```python
from build123d import *

# Parameters (mm, degrees)
BOSS_EXTRUDE1_DEPTH = 4
SKETCH2_R           = 0.2
CUT_EXTRUDE1_DEPTH  = 8
FILLET2_R           = 0.4
FILLET1_R           = 0.6
FILLET3_R           = 2
BOSS_EXTRUDE2_DEPTH = 8
FILLET4_R           = 0.6
CUT_EXTRUDE2_DEPTH  = 0.5
CUT_EXTRUDE2_DRAFT  = -45
CHAMFER1_SIZE       = 0.3


with BuildPart() as part:
    # Sketch1 → Boss-Extrude1 (new, symmetric)
    with BuildSketch(Plane.XY):
        Polygon((0, 9), (6, 9), (6, 0), (7.5, 0), (7.5, -7), (10.5, -7), (10.5, 12), (0, 12), align=None)
    extrude(amount=BOSS_EXTRUDE1_DEPTH, both=True)

    # Sketch2 → Cut-Extrude1 (cut)
    with BuildSketch(Plane.XY.offset(4)):
        with Locations((7.5, -0.2)):
            Circle(SKETCH2_R)
    extrude(amount=-CUT_EXTRUDE1_DEPTH, mode=Mode.SUBTRACT)

    # Fillet2
    fillet2_edges = [part.edges().sort_by_distance(p)[0] for p in [
        (6, 0, 0),
        (7.5, -0.4, 0),
    ]]
    fillet(fillet2_edges, radius=FILLET2_R)

    # Fillet1
    fillet1_edges = [part.edges().sort_by_distance(p)[0] for p in [
        (10.5, -7, 0),
        (7.5, -7, 0),
        (6, 9, 0),
    ]]
    fillet(fillet1_edges, radius=FILLET1_R)

    # Fillet3
    fillet3_edges = [part.edges().sort_by_distance(p)[0] for p in [
        (10.5, 12, 0),
    ]]
    fillet(fillet3_edges, radius=FILLET3_R)

    # Mirror1: part across plane


with BuildPart() as part_1:
    add(part.part)
    add(part.part.mirror(Plane(origin=(0, 12, 4), x_dir=(0, 0, 1), z_dir=(1, 0, 0))))

    # Sketch3 → Boss-Extrude2 (add)
    with BuildSketch(Plane.XY.offset(4)):
        with BuildLine():
            Line((-8.1, -7), (-9.9, -7))
            ThreePointArc((-9.9, -7), (-10.324264069, -6.824264069), (-10.5, -6.4))
            Line((-10.5, -6.4), (-10.5, -10))
            Line((-10.5, -10), (-7.5, -10))
            Line((-7.5, -10), (-7.5, -6.4))
            ThreePointArc((-7.5, -6.4), (-7.675735931, -6.824264069), (-8.1, -7))
        make_face()
    extrude(amount=-BOSS_EXTRUDE2_DEPTH)

    # Fillet4
    fillet4_edges = [part_1.edges().sort_by_distance(p)[0] for p in [
        (-7.5, -10, 0),
    ]]
    fillet(fillet4_edges, radius=FILLET4_R)


with BuildPart() as cut_extrude2_tool:
    # Sketch4 → Cut-Extrude2 (with draft: the straight prism first)
    with BuildSketch(Plane(origin=(0, 12, 0), x_dir=(1, 0, 0), z_dir=(0, 1, 0))):
        Polygon((-2.5, -1.443375673), (2.5, -1.443375673), (0, 2.886751346), align=None)
    extrude(amount=-CUT_EXTRUDE2_DEPTH)
    # Cut-Extrude2: the draft: its side faces are tilted about the plane it starts from
    cut_extrude2_sides = [cut_extrude2_tool.faces().sort_by_distance(p)[0] for p in [
        (0, 11.75, 1.443375673),
        (1.25, 11.75, -0.721687836),
        (-1.25, 11.75, -0.721687836),
    ]]
    draft(cut_extrude2_sides, Plane(origin=(0, 12, 0), x_dir=(1, 0, 0), z_dir=(0, 1, 0)), CUT_EXTRUDE2_DRAFT)


with BuildPart() as part_2:
    add(part_1.part)

    # Cut-Extrude2: cut by cut_extrude2_tool
    add(cut_extrude2_tool.part, mode=Mode.SUBTRACT)

    # Chamfer1
    chamfer1_edges = [part_2.edges().sort_by_distance(p)[0] for p in [
        (-9.3, -10, 4),
        (0, 9, -4),
        (-9.3, -10, -4),
        (-7.675735931, -9.824264069, 4),
        (-7.675735931, -9.824264069, -4),
        (6.95, 0, -4),
        (6.95, 0, 4),
        (7.5, -3.523606798, -4),
        (7.686834472, -0.128635582, -4),
        (7.534851628, -0.483914279, -4),
        (6.117157288, 0.117157288, -4),
        (7.686834472, -0.128635582, 4),
        (7.5, -3.523606798, 4),
        (7.534851628, -0.483914279, 4),
        (6.117157288, 0.117157288, 4),
        (10.5, 1.8, -4),
        (10.5, 1.8, 4),
        (6, 4.4, -4),
        (9, -7, -4),
        (7.675735931, -6.824264069, -4),
        (10.324264069, -6.824264069, -4),
        (9, -7, 4),
        (6, 4.4, 4),
        (7.675735931, -6.824264069, 4),
        (10.324264069, -6.824264069, 4),
        (5.824264069, 8.824264069, -4),
        (5.824264069, 8.824264069, 4),
        (0, 12, -4),
        (0, 12, 4),
        (9.914213562, 11.414213562, -4),
        (9.914213562, 11.414213562, 4),
        (-6, 4.4, 4),
        (-6.95, 0, 4),
        (-7.5, -5.023606798, 4),
        (-10.5, 0, 4),
        (-7.686834472, -0.128635582, 4),
        (-6, 4.4, -4),
        (-6.95, 0, -4),
        (-7.5, -5.023606798, -4),
        (-10.5, 0, -4),
        (-7.686834472, -0.128635582, -4),
        (-6.117157288, 0.117157288, 4),
        (-6.117157288, 0.117157288, -4),
        (-7.534851628, -0.483914279, 4),
        (-7.534851628, -0.483914279, -4),
        (-5.824264069, 8.824264069, 4),
        (-5.824264069, 8.824264069, -4),
        (-9.914213562, 11.414213562, 4),
        (-9.914213562, 11.414213562, -4),
        (0, 9, 4),
    ]]
    chamfer(chamfer1_edges, length=CHAMFER1_SIZE)


solid = part_2.part
```
Could you check a few things on this model? Use its own coordinates, in mm. A direction names the side the tool comes from. Give positions to 0.01 mm unless a question says otherwise; leave off trailing zeros. Write each loop counter-clockwise with the first axis right and the second up, starting at its lowest first coordinate (ties: lowest second). Pieces come first, ordered by that corner, then holes. Notation, with made-up numbers: (-31, 28.5) -> (15, 28.5) arc R12 ccw to (15, 45.5) -> close; hole circle Ø1 at (72, -10.75). An arc over 180 degrees is marked (long way). Write each question's results on one line, items separated by ' | '.
1. Will these pins go through, and if not, where does the flat tip stop? pin 1 Ø2 at (x, z) = (8.5, 1) entering from -Y; pin 2 Ø5 at (x, y) = (-1.5, 4.5) entering from -Z; pin 3 Ø1.2 at (x, z) = (6.5, 0.5) entering from -Y; pin 4 Ø1.4 at (x, z) = (0.5, -0.5) entering from +Y.
Check sheet entries:
pin 1: stops at y = -7 | pin 2: passes through | pin 3: stops at y = 0 | pin 4: stops at y = 11.94
2. I need wall thicknesses on L1, parallel to X at y = -3.75, z = 2.25; L2, parallel to X at y = 6.5, z = -1.75; L3, parallel to Y at x = 4, z = -0.75. Which ranges of each line are inside material? Lowest first, please.
Check sheet entries:
L1: x = -10.5 to -7.5, 7.5 to 10.5 | L2: x = -10.5 to -6, 6 to 10.5 | L3: y = 9 to 12
3. I want a section at A-A, the plane y = 3.5. Write out the boundary of the cut face in (x, z).
Check sheet entries:
outline: (-10.5, -3.7) -> (-10.2, -4) -> (-6.3, -4) -> (-6, -3.7) -> (-6, 3.7) -> (-6.3, 4) -> (-10.2, 4) -> (-10.5, 3.7) -> close; (6, -3.7) -> (6.3, -4) -> (10.2, -4) -> (10.5, -3.7) -> (10.5, 3.7) -> (10.2, 4) -> (6.3, 4) -> (6, 3.7) -> close
4. I want a section at D-D, the plane y = -3.25. Write out the boundary of the cut face in (x, z).
Check sheet entries:
outline: (-10.5, -3.7) -> (-10.2, -4) -> (-7.8, -4) -> (-7.5, -3.7) -> (-7.5, 3.7) -> (-7.8, 4) -> (-10.2, 4) -> (-10.5, 3.7) -> close; (7.5, -3.7) -> (7.8, -4) -> (10.2, -4) -> (10.5, -3.7) -> (10.5, 3.7) -> (10.2, 4) -> (7.8, 4) -> (7.5, 3.7) -> close
5. If we mould it in two halves opening along Z, with no side actions, what happens to faces 1 (the conical face through (5.9, 8.911, -3.815)), 2 (the flat face through (0, 12, 2)), 3 (the flat face through (-1.019, 11.754, -0.629)), 4 (the flat face through (1.05, 11.75, -0.57))? For each: released by +Z, released by -Z, zero draft, split by the parting line, or undercut.
Check sheet entries:
face 1: released by -Z | face 2: zero draft | face 3: undercut | face 4: undercut
6. I want a section at C-C, the plane x = -1. Write out the boundary of the cut face in (y, z).
Check sheet entries:
outline: (9, -3.7) -> (9.3, -4) -> (11.7, -4) -> (12, -3.7) -> (12, -1.15) -> (11.5, -0.15) -> (11.5, 0.94) -> (12, 1.44) -> (12, 3.7) -> (11.7, 4) -> (9.3, 4) -> (9, 3.7) -> close
7. On a 3-axis mill with a long thin cutter (end or side, diameter ignored), from which of +Z, -Z, +X, -X, +Y, -Y can I reach the whole of each face in a straight line? I mean faces 5 (the conical face through (-5.914, 8.903, 3.819)), 6 (the flat face through (10.5, 2, 0)), 7 (the flat face through (7.5, -3, 0)), 8 (the flat face through (9, -7, 0)). Say none if no direction works.
Check sheet entries:
face 5: +Z, -Y | face 6: +Z, -Z, +X, +Y, -Y | face 7: +Z, -Z, -Y | face 8: +Z, -Z, +X, -Y
8. I want a section at B-B, the plane z = 2. Write out the boundary of the cut face in (x, y).
Check sheet entries:
outline: (-10.5, -10) -> (-8.1, -10) arc R0.6 ccw to (-7.5, -9.4) -> (-7.5, -0.65) arc R0.4 ccw to (-7.63, -0.35) arc R0.2 cw to (-7.5, 0) -> (-6.4, 0) arc R0.4 ccw to (-6, 0.4) -> (-6, 8.4) arc R0.6 cw to (-5.4, 9) -> (5.4, 9) arc R0.6 cw to (6, 8.4) -> (6, 0.4) arc R0.4 ccw to (6.4, 0) -> (7.5, 0) arc R0.2 cw to (7.63, -0.35) arc R0.4 ccw to (7.5, -0.65) -> (7.5, -6.4) arc R0.6 ccw to (8.1, -7) -> (9.9, -7) arc R0.6 ccw to (10.5, -6.4) -> (10.5, 10) arc R2 ccw to (8.5, 12) -> (-8.5, 12) arc R2 ccw to (-10.5, 10) -> close
